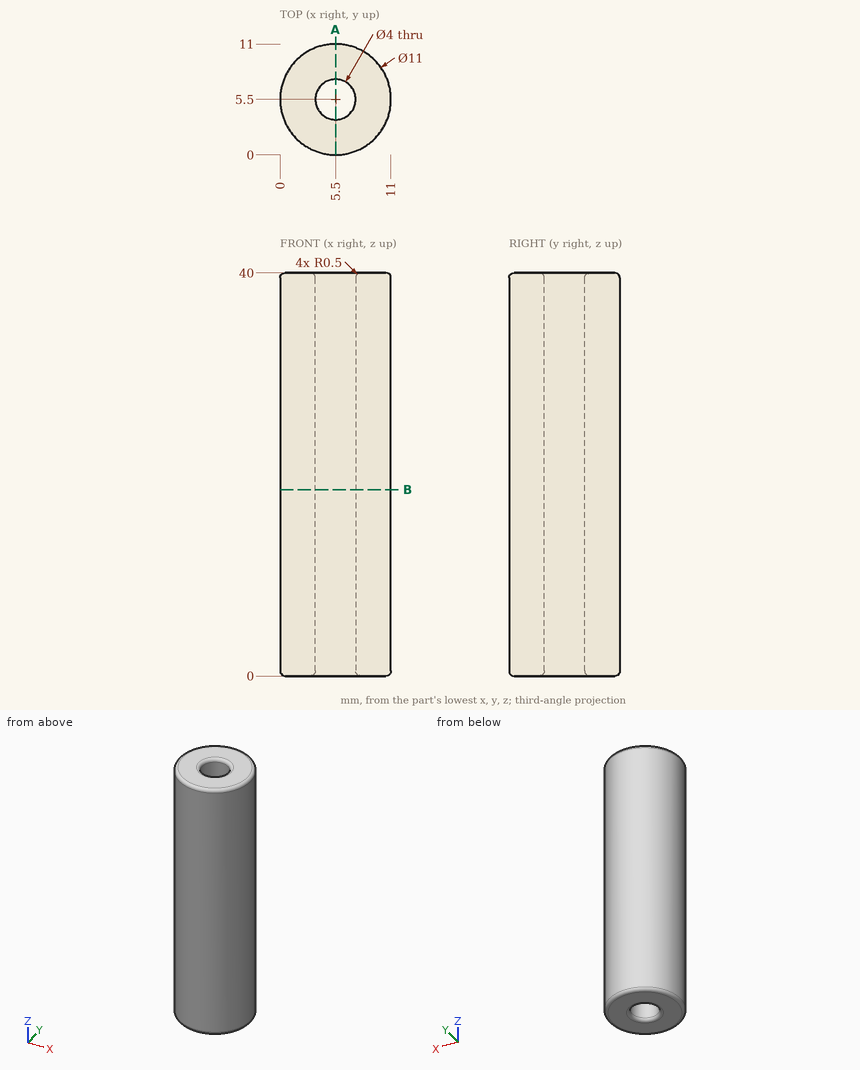
Check sheet for the drawn part. Datum: minimum x, y, z corner. Units: mm. Give positions to 0.01 mm unless a question says otherwise; leave off trailing zeros. Order: outer loops, then holes, each group sorted by start corner. A loop starts at its lowest first (then second) coordinate and runs counter-clockwise, first axis right, second up. Notation, with made-up numbers: (-14.5, 28) -> (14.5, 28) arc R22 ccw to (14.5, 55) -> close; hole circle Ø5 at (-5, 65.25). An arc over 180 degrees is marked (long way). One line per item, written item: value.
(1) Gauge pin test, flat end, axial feed: pin 1 (1.5 mm diameter, centred on x = 7, z = 34, fed in from -Y). Record the tip position at first contact, or that the pin passes through.
Final values:
pin 1: y = 0.05
(2) Sectioned sample at A-A on x = 5.5. Record the cut outline in (y, z), then the cut area to 3 significant figures.
Final values:
outline: (0, 0.5) arc R0.5 ccw to (0.5, 0) -> (3, 0) arc R0.5 ccw to (3.5, 0.5) -> (3.5, 39.5) arc R0.5 ccw to (3, 40) -> (0.5, 40) arc R0.5 ccw to (0, 39.5) -> close; (7.5, 0.5) arc R0.5 ccw to (8, 0) -> (10.5, 0) arc R0.5 ccw to (11, 0.5) -> (11, 39.5) arc R0.5 ccw to (10.5, 40) -> (8, 40) arc R0.5 ccw to (7.5, 39.5) -> close
area: 280 mm^2
(3) Scan lines: line 1 along Y through (x, z) = (5.5, 14.5); line 2 along Y through (x, z) = (5, 38); line 3 along X through (y, z) = (4.5, 37.5). Record each from-to range of solid material in increasing order. Write a range as [from, to].
Final values:
line 1: [0, 3.5], [7.5, 11]
line 2: [0.02, 3.56], [7.44, 10.98]
line 3: [0.09, 3.77], [7.23, 10.91]
(4) Sectioned sample at B-B on z = 18.5. Record the cut outline in (x, y), then the cut area to 3 significant figures.
Final values:
outline: circle Ø11 at (5.5, 5.5); hole circle Ø4 at (5.5, 5.5)
area: 82.5 mm^2
